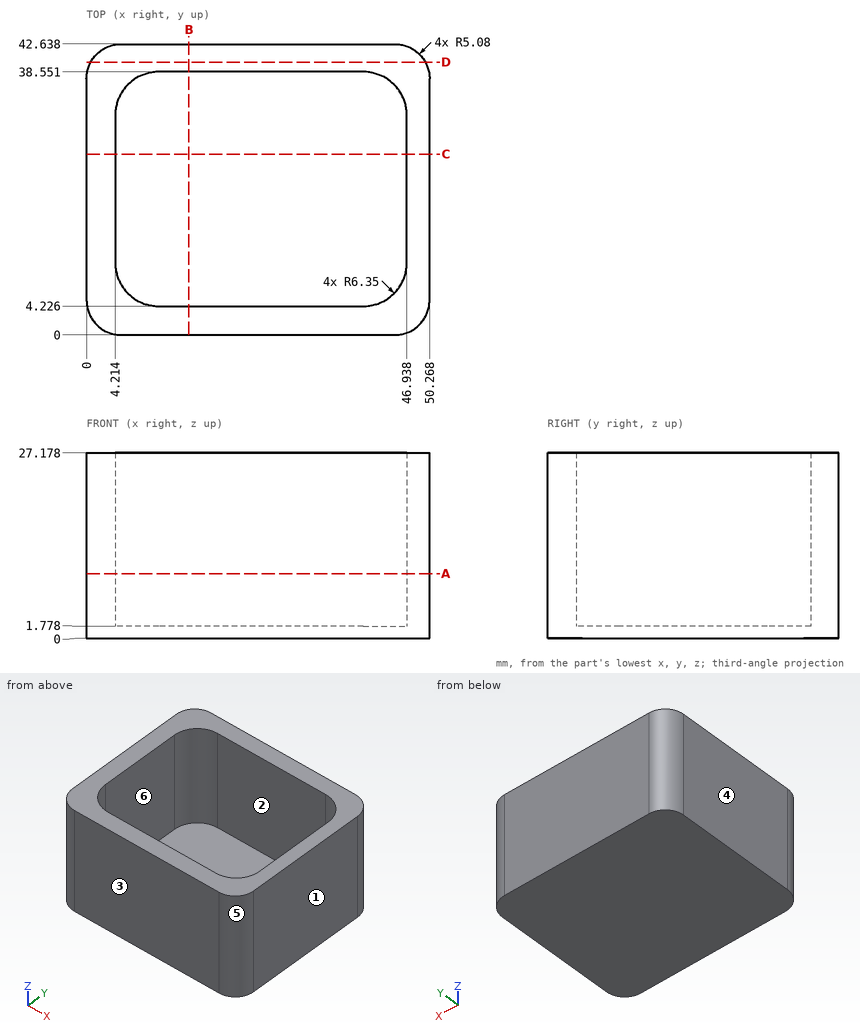
Print and shaded views of the part. All mm, measured from the part's lowest x, y and z. A direction names the side the tool comes from. Give positions to 0.01 mm unless a question says otherwise; leave off trailing zeros. Write each loop counter-clockwise with the first axis right and the second up, starting at its lowest first coordinate (ties: lowest second). Pieces come first, ordered by that corner, then holes. Notation, with made-up numbers: (-37.75, 28) -> (-4.75, 28) arc R3 cw to (-4.75, 32) -> close; hole circle Ø8 at (25, -25.75). An arc over 180 degrees is marked (long way). Use CSV: the item, a comma, the result in double quotes. Start each with the question number.
1) Tool access for the marked faces 5 and 6: list every direction of +Z, -Z, +X, -X, +Y, -Y with a clear straight run to the whole face (end or side of a thin tool).
2) Cut at C-C on y = 26.5. List the corners of the cut face in (x, z), plus the area to 3 significant figures.
3) Cut at A-A on z = 9.5. List the corners of the cut face in (x, y), plus the area to 3 significant figures.
4) Cut at B-B on x = 15. List the corners of the cut face in (y, z), plus the area to 3 significant figures.
5) Two-plate mould, pull along X, no slides. Class the marked faces 1, 2, 3 and 4: released by +X, released by -X, zero draft, split by the parting line, or undercut.
6) Drill centre lines: L1, parallel to Y at x = 36, z = 13.5; L2, parallel to X at y = 22, z = 12.5; L3, parallel to Z at x = 42, y = 29. Where is each one in solid material? Low to high.
7) Cut at D-D on y = 40. List the corners of the cut face in (x, z).
8) Pin check, flat tips, straight feed: P1, Ø2, axis at y = 29, z = 16.5, coming from the -X side; P2, Ø17, axis at x = 36, y = 15.5, coming from the +Z side. Stop position of each tip, or through.
Final values:
1,face 5,"+Z, -Z, +X, -Y"
1,face 6,"+Z"
2,outline,"(0, 0) -> (50.27, 0) -> (50.27, 27.18) -> (46.94, 27.18) -> (46.94, 1.78) -> (4.21, 1.78) -> (4.21, 27.18) -> (0, 27.18) -> close"
2,area,"281 mm2"
3,outline,"(0, 5.08) arc R5.08 ccw to (5.08, 0) -> (45.19, 0) arc R5.08 ccw to (50.27, 5.08) -> (50.27, 37.56) arc R5.08 ccw to (45.19, 42.64) -> (5.08, 42.64) arc R5.08 ccw to (0, 37.56) -> close; hole (4.21, 10.58) arc R6.35 ccw to (10.56, 4.23) -> (40.59, 4.23) arc R6.35 ccw to (46.94, 10.58) -> (46.94, 32.2) arc R6.35 ccw to (40.59, 38.55) -> (10.56, 38.55) arc R6.35 ccw to (4.21, 32.2) -> close"
3,area,"689 mm2"
4,outline,"(0, 0) -> (42.64, 0) -> (42.64, 27.18) -> (38.55, 27.18) -> (38.55, 1.78) -> (4.23, 1.78) -> (4.23, 27.18) -> (0, 27.18) -> close"
4,area,"287 mm2"
5,face 1,"released by +X"
5,face 2,"undercut"
5,face 3,"zero draft"
5,face 4,"released by -X"
6,L1,"y = 0 to 4.23, 38.55 to 42.64"
6,L2,"x = 0 to 4.21, 46.94 to 50.27"
6,L3,"z = 0 to 1.78"
7,outline,"(0.63, 0) -> (49.64, 0) -> (49.64, 27.18) -> (0.63, 27.18) -> close"
8,P1,"stops at x = 0"
8,P2,"stops at z = 1.78"
